Could you check a few things on this model? Use its own coordinates, in mm. Face numbers are marked on the shaded views. Round coordinates to 2 decimals unless told otherwise and drop trailing zeros. Write each loop counter-clockwise with the first axis right and the second up, starting at its lowest first coordinate (ties: lowest second). Pieces come first, ordered by that corner, then holes. Notation, with made-up numbers: (59.5, 2.5) -> (102.5, 2.5) arc R10 cw to (102.5, 7.5) -> close; hole circle Ø10 at (-25.75, 53.5). An arc over 180 degrees is marked (long way). Return JSON: item names as keys, results as strings.
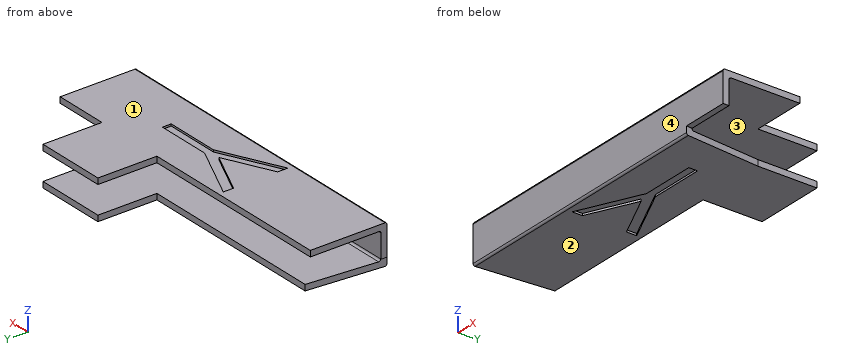
from build123d import *

# Parameters (mm, degrees)
IZIM1_W                     = 70
IZIM1_H                     = 19.5
Y_KSEKLIK_EKSTR_ZYON1_DEPTH = 10
BO_ALTMA1_T                 = -1.5
RADYUS1_R                   = 0.5
RADYUS2_R                   = 0.5
KES_EKSTR_ZYON1_DEPTH       = 2
Y_KSEKLIK_EKSTR_ZYON3_DEPTH = 10
IZIM8_W                     = 18
IZIM8_H                     = 1.5
Y_KSEKLIK_EKSTR_ZYON4_DEPTH = 15
KES_EKSTR_ZYON3_DEPTH       = 10
IZIM10_W                    = 1.5
IZIM10_H                    = 15
KES_EKSTR_ZYON4_DEPTH       = 18
KES_EKSTR_ZYON5_DEPTH       = 0.5
Y_KSEKLIK_EKSTR_ZYON5_DEPTH = 2


with BuildPart() as part:
    # Çizim1 → Yükseklik-Ekstrüzyon1 (new body)
    with BuildSketch(Plane.XY):
        Rectangle(IZIM1_W, IZIM1_H)
    extrude(amount=Y_KSEKLIK_EKSTR_ZYON1_DEPTH)

    # İç Boşaltma1
    bo_altma1_openings = [part.faces().sort_by_distance(p)[0] for p in [
        (-35, 0, 5),
        (0, 9.75, 5),
        (35, 0, 5),
    ]]
    offset(amount=BO_ALTMA1_T, openings=bo_altma1_openings, kind=Kind.INTERSECTION)

    # Radyus1
    radyus1_edges = [part.edges().sort_by_distance(p)[0] for p in [
        (0, -8.25, 1.5),
        (0, -8.25, 8.5),
    ]]
    fillet(radyus1_edges, radius=RADYUS1_R)

    # Radyus2
    radyus2_edges = [part.edges().sort_by_distance(p)[0] for p in [
        (0, -9.75, 10),
        (0, -9.75, 0),
    ]]
    fillet(radyus2_edges, radius=RADYUS2_R)

    # Çizim2 → Kes-Ekstrüzyon1 (cut)
    with BuildSketch(Plane(origin=(0, 0, 0), x_dir=(-1, 0, 0), z_dir=(0, 0, -1))):
        Polygon((35, -9.75), (33.293971061, 9.75), (35, 9.75), align=None)
    kes_ekstr_zyon1 = extrude(amount=-KES_EKSTR_ZYON1_DEPTH, mode=Mode.SUBTRACT)

    # Aynalama1: Kes-Ekstrüzyon1 across plane
    add(kes_ekstr_zyon1.mirror(Plane(origin=(0, 0, 0), x_dir=(0, 0, 1), z_dir=(1, 0, 0))), mode=Mode.SUBTRACT)

    # Çizim7 → Yükseklik-Ekstrüzyon3 (add)
    with BuildSketch(Plane.ZY.offset(35)):
        with BuildLine():
            Line((2, -8.25), (2, -9.75))
            Line((2, -9.75), (9.5, -9.75))
            ThreePointArc((9.5, -9.75), (9.853553391, -9.603553391), (10, -9.25))
            Line((10, -9.25), (10, 9.75))
            Line((10, 9.75), (8.5, 9.75))
            Line((8.5, 9.75), (8.5, -7.75))
            ThreePointArc((8.5, -7.75), (8.353553391, -8.103553391), (8, -8.25))
            Line((8, -8.25), (2, -8.25))
        make_face()
    y_kseklik_ekstr_zyon3 = extrude(amount=Y_KSEKLIK_EKSTR_ZYON3_DEPTH)

    # Çizim8 → Yükseklik-Ekstrüzyon4 (add)
    with BuildSketch(Plane(origin=(0, 9.75, 0), x_dir=(1, 0, 0), z_dir=(0, 1, 0))):
        with Locations((-24.293971061, -0.75)):
            Rectangle(IZIM8_W, IZIM8_H)
        with Locations((-24.293971061, -9.25)):
            Rectangle(IZIM8_W, IZIM8_H)
    y_kseklik_ekstr_zyon4 = extrude(amount=Y_KSEKLIK_EKSTR_ZYON4_DEPTH)

    # Aynalama3: Yükseklik-Ekstrüzyon3, Yükseklik-Ekstrüzyon4 across plane
    add(y_kseklik_ekstr_zyon3.mirror(Plane(origin=(0, 0, 0), x_dir=(0, 0, 1), z_dir=(1, 0, 0))))
    add(y_kseklik_ekstr_zyon4.mirror(Plane(origin=(0, 0, 0), x_dir=(0, 0, 1), z_dir=(1, 0, 0))))

    # Çizim9 → Kes-Ekstrüzyon3 (cut)
    with BuildSketch(Plane.ZY.offset(45)):
        with BuildLine():
            Line((2, -9.75), (9.5, -9.75))
            ThreePointArc((9.5, -9.75), (9.853553391, -9.603553391), (10, -9.25))
            Line((10, -9.25), (10, 9.75))
            Line((10, 9.75), (8.5, 9.75))
            Line((8.5, 9.75), (8.5, -7.75))
            ThreePointArc((8.5, -7.75), (8.353553391, -8.103553391), (8, -8.25))
            Line((8, -8.25), (2, -8.25))
            Line((2, -8.25), (2, -9.75))
        make_face()
    extrude(amount=-KES_EKSTR_ZYON3_DEPTH, mode=Mode.SUBTRACT)

    # Çizim10 → Kes-Ekstrüzyon4 (cut)
    with BuildSketch(Plane.ZY.offset(33.293971061)):
        with Locations((0.75, 17.25)):
            Rectangle(IZIM10_W, IZIM10_H)
        with Locations((9.25, 17.25)):
            Rectangle(IZIM10_W, IZIM10_H)
    extrude(amount=-KES_EKSTR_ZYON4_DEPTH, mode=Mode.SUBTRACT)

    # Çizim11 → Kes-Ekstrüzyon5 (cut)
    with BuildSketch(Plane.XY.offset(10)):
        Polygon((-4.810195605, 8.458867521), (-4.810195605, 5.846955128), (7.246578567, 0.25), (-4.810195605, -5.346955128), (-4.810195605, -7.958867521), (10.458997604, -0.869391026), (24.293971061, -0.869391026), (24.293971061, 1.369391026), (10.458997604, 1.369391026), align=None)
    kes_ekstr_zyon5 = extrude(amount=-KES_EKSTR_ZYON5_DEPTH, mode=Mode.SUBTRACT)

    # Aynalama4: Kes-Ekstrüzyon5 across plane
    add(kes_ekstr_zyon5.mirror(Plane.XY.offset(5)), mode=Mode.SUBTRACT)

    # Çizim12 → Yükseklik-Ekstrüzyon5 (add)
    with BuildSketch(Plane(origin=(45, 0, 0), x_dir=(0, 0, -1), z_dir=(1, 0, 0))):
        with BuildLine():
            Line((-9.5, -9.75), (-2, -9.75))
            Line((-2, -9.75), (-2, -8.25))
            Line((-2, -8.25), (-8, -8.25))
            ThreePointArc((-8, -8.25), (-8.353553391, -8.103553391), (-8.5, -7.75))
            Line((-8.5, -7.75), (-8.5, 9.75))
            Line((-8.5, 9.75), (-10, 9.75))
            Line((-10, 9.75), (-10, -9.25))
            ThreePointArc((-10, -9.25), (-9.853553391, -9.603553391), (-9.5, -9.75))
        make_face()
    extrude(amount=Y_KSEKLIK_EKSTR_ZYON5_DEPTH)


solid = part.part
1) I want a section at D-D, the plane y = 3.5. Please give me the cut outline in (x, z).
Return value:
{"outline": "(-35, 8.5) -> (47, 8.5) -> (47, 10) -> (5.87, 10) -> (5.87, 9.5) -> (0.25, 9.5) -> (0.25, 10) -> (-35, 10) -> close; (-33.84, 0) -> (0.25, 0) -> (0.25, 0.5) -> (5.87, 0.5) -> (5.87, 0) -> (33.84, 0) -> (33.84, 1.5) -> (-33.84, 1.5) -> close"}
2) Will these pins go through, and if not, where does the flat tip stop? pin 1 Ø1.6 at (y, z) = (18, 9.5) entering from +X; pin 2 Ø0.6 at (x, z) = (16, 10) entering from -Y; pin 3 Ø1 at (x, z) = (38.5, 5) entering from +Y.
Return value:
{"pin 1": "x = 33.29", "pin 2": "y = -9.71", "pin 3": "y = -8.25"}
3) I want a section at C-C, the plane z = 5. Please give me the cut outline in (x, y), and give its area (3 significant figures).
Return value:
{"outline": "(-35, -9.75) -> (47, -9.75) -> (47, -8.25) -> (-35, -8.25) -> close", "area": "123 mm²"}
4) Thinking about a two-plate mould opening in Z: for the marked faces 1, 2, 3 and 4, which applies, pulls with the +Z half, pulls with the -Z half, needs draft (parallel to the pull), parting line crosses it, or undercut?
Return value:
{"face 1": "pulls with the +Z half", "face 2": "pulls with the -Z half", "face 3": "undercut", "face 4": "needs draft"}
5) I want a section at A-A, the plane y = 19.5. Please give me the cut outline in (x, z), and give its area (3 significant figures).
Return value:
{"outline": "(15.29, 0) -> (33.29, 0) -> (33.29, 1.5) -> (15.29, 1.5) -> close; (15.29, 8.5) -> (33.29, 8.5) -> (33.29, 10) -> (15.29, 10) -> close", "area": "54.0 mm²"}
6) I want a section at B-B, the plane x = -8. Please give me the cut outline in (y, z), and give its area (3 significant figures).
Return value:
{"outline": "(-9.75, 0.5) arc R0.5 ccw to (-9.25, 0) -> (9.75, 0) -> (9.75, 1.5) -> (-7.75, 1.5) arc R0.5 cw to (-8.25, 2) -> (-8.25, 8) arc R0.5 cw to (-7.75, 8.5) -> (9.75, 8.5) -> (9.75, 10) -> (-9.25, 10) arc R0.5 ccw to (-9.75, 9.5) -> close", "area": "69.0 mm²"}
7) If I drill on probe 1 along Z at (x, y) = (-6, 4.5); probe 2 along Z at (x, y) = (14, 1); probe 3 along Y at (x, z) = (-27, 3), over which ranges is the centre line in solid material (lowest first)? Write a range as [from, to].
Return value:
{"probe 1": "[0, 1.5], [8.5, 10]", "probe 2": "[0.5, 1.5], [8.5, 9.5]", "probe 3": "[-9.75, -8.25]"}
